For this review, take the finished solid that the model builds, in its own axes (mm). A direction names the side the tool comes from. Give positions to 0.01 mm unless a question says otherwise; leave off trailing zeros. Write each loop counter-clockwise with the first axis right and the second up, starting at its lowest first coordinate (ties: lowest second). Pieces come first, ordered by that corner, then holes.
Autodesk Inventor part; units mm, degrees
ref_plane "YZ Plane" through (0, 0, 0) normal (1, 0, 0) x (0, 1, 0)
ref_plane "XZ Plane" through (0, 0, 0) normal (0, 1, 0) x (-1, 0, 0)
ref_plane "XY Plane" through (0, 0, 0) normal (0, 0, 1) x (1, 0, 0)
sketch "Sketch1" plane through (0, 0, 0) normal (0, 1, 0) x (-1, 0, 0)
  line L0 (3.9616, -0.4601) -> (4.9616, -0.4601)
  line L1 (5.4616, 1.5399) -> (7.4616, 1.5399)
  line L2 (7.4616, 1.5399) -> (7.4616, -10.4601)
  line L3 (7.4616, -10.4601) -> (5.4616, -10.4601)
  line L4 (4.9616, -8.4601) -> (3.9616, -8.4601)
  line L5 (5.4616, 1.5399) -> (4.9616, -0.4601)
  line L6 (3.4616, 1.5399) -> (3.9616, -0.4601)
  line L7 (4.9616, -8.4601) -> (5.4616, -10.4601)
  line L8 (3.4616, -10.4601) -> (3.9616, -8.4601)
  line L9 (3.4616, -10.4601) -> (3.4616, -17.9601)
  line L10 (3.4616, -17.9601) -> (12.9616, -17.9601)
  line L11 (12.9616, -17.9601) -> (12.9616, 9.0399)
  line L12 (12.9616, 9.0399) -> (3.4616, 9.0399)
  line L13 (3.4616, 9.0399) -> (3.4616, 1.5399)
  point P0 (0, 0)
  point P1 (12.9616, -4.4601)
  point P2 (7.4616, -4.4601)
  point P3 (6.4616, -10.4601)
  dimension "d2" = 8
  dimension "d3" = 1
  dimension "d5" = 0.5
  dimension "d6" = 4
  dimension "d8" = 9.5
  dimension "d9" = 27
  dimension "d12" = 0
  dimension "d13" = 12
  dimension "d14" = 2
  dimension "d15" = 2
extrude "Extrusion1" add sketch "Sketch1" along normal blind 35.25
sketch "Sketch2" plane through (-12.9616, 0, -17.9601) normal (-1, 0, 0) x (0, 0, 1)
  line L0 (0, 35.25) -> (27, 35.25)
  line L1 (0, 0) -> (0, 35.25)
  point P0 (17.9601, 0)
  point P1 (3.5, 25.125)
  point P2 (23.5, 25.125)
  point P3 (23.5, 10.125)
  point P4 (3.5, 10.125)
  dimension "d16" = 20
  dimension "d17" = 20
  dimension "d18" = 15
  dimension "d19" = 15
  dimension "d20" = 0
  dimension "d21" = 0
  dimension "d22" = 35.25
  dimension "d23" = 27
  dimension "d24" = 10.125
  dimension "d25" = 3.5
hole "Hole1" at (-12.9616, 25.125, -14.4601) at (-12.9616, 25.125, 5.5399) at (-12.9616, 10.125, 5.5399) at (-12.9616, 10.125, -14.4601) direction (1, 0, 0) diameter 2.459 depth 5 tip angle 118
sketch "Sketch3" plane through (-12.9616, 0, -17.9601) normal (-1, 0, 0) x (0, 0, 1)
  line L0 (0, 35.25) -> (27, 35.25)
  line L1 (0, 0) -> (0, 35.25)
  line L2 (27, 35.25) -> (0, 35.25)
  line L3 (0, 35.25) -> (0, 28.575)
  line L4 (0, 28.575) -> (27, 28.575)
  line L5 (27, 28.575) -> (27, 35.25)
  line L6 (27, 0) -> (0, 0)
  line L7 (0, 0) -> (0, 6.675)
  line L8 (0, 6.675) -> (27, 6.675)
  line L9 (27, 6.675) -> (27, 0)
  point P0 (17.9601, 0)
  point P1 (0, 6.675)
  dimension "d33" = 35.25
  dimension "d34" = 21.9
  dimension "d35" = 6.675
extrude "Extrusion2" cut sketch "Sketch3" against normal blind 0.5
equation "\"d35\" = -0.5 * d34 + 0.5 * d33"
equation "\"GapSize\" = Thickness"
equation "\"BendRadius\" = Thickness"
equation "\"MinimumRemnant\" = 2 * Thickness"
equation "\"BendReliefDepth\" = 0.5 * Thickness"
equation "\"BendReliefWidth\" = Thickness"
equation "\"CornerReliefSize\" = 4 * Thickness"
equation "\"JacobiRadiusSize\" = BendRadius"
equation "\"TransitionRadius\" = BendRadius"
properties part number "Guia do trilho" material "Steel, Alloy"
(1) We need section B-B (y = 17). Write out the cut boundary in (x, z).
(2) The part is to be moulded in two halves that separate along X. For faces 1 (the flat face through (-12.462, 3, -5)), 2 (the cylindrical face through (-10.427, 26.325, 5.273)), 3 (the flat face through (-5.215, 17.378, 0.554)), say which applies: +X half, -X half, draft (parallel to the pull), parting line (faces both ways), or undercut.
(3) Tool access review of faces 4 (the flat face through (-6, 17, -10.46)), 5 (the flat face through (-4.5, 17.4, -0.46)), 6 (the cylindrical face through (-10.43, 10.87, 4.56)): name each direction out of +Z, -Z, +X, -X, +Y, -Y from which nothing blocks a thin tool from reaching the whole face with its end or side.
(4) We need section A-A (x = -6). Write out the cut boundary in (y, z).
(5) We need section D-D (x = -9.25). Count the separate pieces of the cut face and the enclosed holes in it, and give its area (3 significant figures).
(6) Clearance check with flat-ended pins moving along their axes: pin 1 Ø2 at (x, z) = (-11.5, -3.5) entering from -Y; pin 2 Ø2 at (y, z) = (5, -4.5) entering from -X; pin 3 Ø2 at (y, z) = (10.12, -14.46) entering from -X; pin 4 Ø3.5 at (y, z) = (19, -2.5) entering from +X. State where each tip first meets the part, or that it passes through.
(7) For L1, parallel to Y at x = -8.5, z = -13.75; L2, parallel to Z at x = -6.75, y = 22; L3, parallel to Z at x = -4, y = 5.5, list the stretches that pass through material, from the lowest coordinate up.
(8) We need section C-C (z = 1). Write out the cut boundary in (x, y) (3 decimals), and give its area (3 significant figures).
The answers:
1. outline: (-12.96, -17.96) - (-3.46, -17.96) - (-3.46, -10.46) - (-3.96, -8.46) - (-4.96, -8.46) - (-5.46, -10.46) - (-7.46, -10.46) - (-7.46, 1.54) - (-5.46, 1.54) - (-4.96, -0.46) - (-3.96, -0.46) - (-3.46, 1.54) - (-3.46, 9.04) - (-12.96, 9.04) - close
2. face 1: -X half
2. face 2: draft
2. face 3: undercut
3. face 4: +Y, -Y
3. face 5: +X, +Y, -Y
3. face 6: -X
4. outline: (0, -17.96) - (35.25, -17.96) - (35.25, -10.46) - (0, -10.46) - close; (0, 1.54) - (35.25, 1.54) - (35.25, 9.04) - (0, 9.04) - close
5. separate pieces: 1
5. enclosed holes: 4
5. area: 933 mm2
6. pin 1: stops at y = 0
6. pin 2: stops at x = -12.46
6. pin 3: stops at x = -7.83
6. pin 4: stops at x = -7.46
7. L1: y = 0 to 9.12, 11.13 to 24.12, 26.13 to 35.25
7. L2: z = -17.96 to -10.46, 1.54 to 9.04
7. L3: z = -17.96 to -8.46, -0.46 to 9.04
8. outline: (-12.962, 6.675) - (-12.462, 6.675) - (-12.462, 0) - (-7.462, 0) - (-7.462, 35.25) - (-12.462, 35.25) - (-12.462, 28.575) - (-12.962, 28.575) - close; (-5.327, 0) - (-3.597, 0) - (-3.597, 35.25) - (-5.327, 35.25) - close
8. area: 248 mm2
